Verification items for this drawing (mm, ordinates from the low corner). A direction names the side the tool comes from. Coordinates: 2 decimals unless noted, no trailing zeros. Loops run counter-clockwise (first coordinate to the right, second up) from the corner with the lowest first, then second, coordinate; pieces in that order, holes last. Notation, with made-up numbers: (-1, 60.5) -> (21, 60.5) arc R10 ccw to (21, 72.5) -> close; hole circle Ø10 at (86, -1.75). An arc over 180 degrees is marked (long way). Write item = value, one per line.
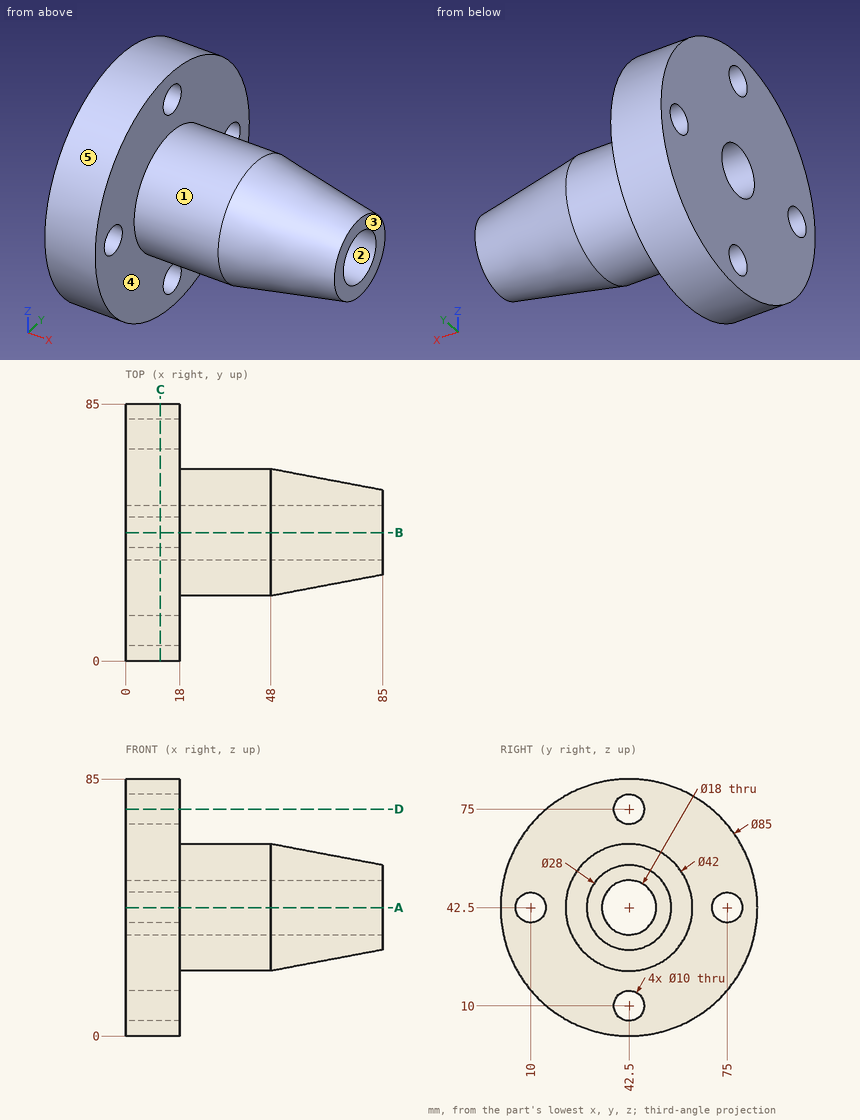
1) Depth check by flat-ended pin: pin 1 Ø6 at (y, z) = (42.5, 75) entering from +X; pin 2 Ø1.5 at (x, y) = (75, 29.5) entering from -Z; pin 3 Ø10 at (y, z) = (58, 17.5) entering from -X; pin 4 Ø10 at (x, y) = (47.5, 35.5) entering from -Z. Enter the tip coordinate at first touch or a pass-through.
Ans:
pin_1 = through
pin_2 = 32.35
pin_3 = 0
pin_4 = 21.6
2) Release check for a two-part mould opening along Y. For the marked faces 1, 2 and 3 record: pulls with the +Y half, pulls with the -Y half, needs draft (parallel to the pull), parting line crosses it, or undercut.
Ans:
face_1 = parting line crosses it
face_2 = undercut
face_3 = needs draft
3) Sectioned sample at D-D, the plane z = 75. Record the cut outline in (x, y), plus the area to 3 significant figures.
Ans:
outline = (0, 15.11) -> (18, 15.11) -> (18, 37.5) -> (0, 37.5) -> close; (0, 47.5) -> (18, 47.5) -> (18, 69.89) -> (0, 69.89) -> close
area = 806 mm2
4) Material ranges on line 1 (Z direction, x = 9, y = 42.5); line 2 (X direction, y = 54, z = 77.5); line 3 (Y direction, x = 53.5, z = 44), recorded low to high.
Ans:
line_1 = 0 to 5, 15 to 33.5, 51.5 to 70, 80 to 85
line_2 = 0 to 18
line_3 = 22.6 to 33.63, 51.37 to 62.4
5) Sectioned sample at C-C, the plane x = 11.5. Record the cut outline in (y, z), plus the area to 3 significant figures.
Ans:
outline = circle Ø85 at (42.5, 42.5); hole circle Ø10 at (10, 42.5); hole circle Ø18 at (42.5, 42.5); hole circle Ø10 at (42.5, 10); hole circle Ø10 at (42.5, 75); hole circle Ø10 at (75, 42.5)
area = 5,110 mm2
6) Sectioned sample at A-A, the plane z = 42.5. Record the cut outline in (x, y), plus the area to 4 significant figures.
Ans:
outline = (0, 0) -> (18, 0) -> (18, 5) -> (0, 5) -> close; (0, 15) -> (18, 15) -> (18, 21.5) -> (48, 21.5) -> (85, 28.5) -> (85, 33.5) -> (0, 33.5) -> close; (0, 51.5) -> (85, 51.5) -> (85, 56.5) -> (48, 63.5) -> (18, 63.5) -> (18, 70) -> (0, 70) -> close; (0, 80) -> (18, 80) -> (18, 85) -> (0, 85) -> close
area = 2,195 mm2
7) Tool access check on the marked faces 4 and 5. Record the directions out of +Z, -Z, +X, -X, +Y, -Y that give a thin tool (end or side, any length) a straight path to the whole face; none if there is none.
Ans:
face_4 = +X
face_5 = +X, -X
